Print and shaded views of the part. All mm, measured from the part's lowest x, y and z. A direction names the side the tool comes from. Coordinates: 2 decimals unless noted, no trailing zeros. Order: outer loops, then holes, each group sorted by start corner. A loop starts at its lowest first (then second) coordinate and runs counter-clockwise, first axis right, second up. Notation, with made-up numbers: (33.25, -21.75) -> (51.25, -21.75) arc R21 cw to (51.25, 12.25) -> close; hole circle Ø8 at (80, -32). An arc over 180 degrees is marked (long way). Return JSON: item names as keys, results as strings. Group by question number.
1) Cut at C-C (z = 12.75). Write the cut outline in (x, y), and give its area (3 significant figures).
2) Pull direction X, two halves, no side cores. Call the marked faces 1, 2 and 3: +X half, -X half, draft (parallel to the pull), parting line (faces both ways), or undercut.
3) Probe line 1 (Y direction, x = 12, z = 12.6); line 2 (Y direction, x = 11.5, z = 8); line 3 (Z direction, x = 20, y = 3.3). List the from-to ranges inside material, lowest first.
4) Cut at B-B (z = 7). Write the cut outline in (x, y).
5) Cut at A-A (x = 12). Write the cut outline in (y, z).
6) Flat gauge pins, fed straight in: pin 1 (2.5 mm diameter, centred on x = 4.5, z = 6.5, fed in from +Y); pin 2 (1.5 mm diameter, centred on x = 8, y = 6.5, fed in from -Z); pin 3 (1 mm diameter, centred on x = 3.5, y = 4, fed in from -Z). Where does each tip first touch, or does it go through?
7) Cut at D-D (y = 12). Write the cut outline in (x, z).
8) Which spindle directions (+Z, -Z, +X, -X, +Y, -Y) get a long thin tool onto all of the face, cutting with end or side? Do the marked faces 4, 5 and 6. Say none if no direction does.
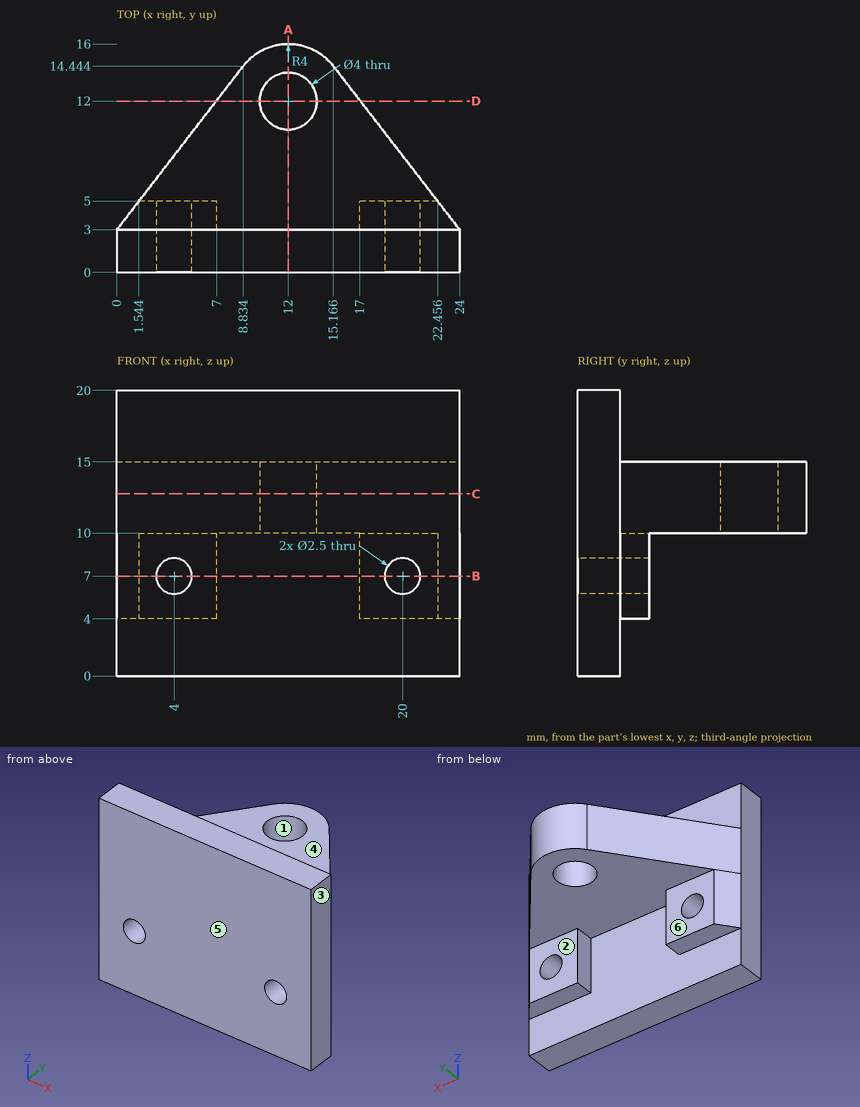
Answers below:
{
 "1": {"outline": "(0, 0) -> (24, 0) -> (24, 3) -> (15.17, 14.44) arc R4 ccw to (8.83, 14.44) -> (0, 3) -> close; hole circle Ø4 at (12, 12)", "area": "240 mm^2"},
 "2": {"face 1": "undercut", "face 2": "draft", "face 3": "+X half"},
 "3": {"line 1": "y = 0 to 10, 14 to 16", "line 2": "y = 0 to 3", "line 3": "z = 4 to 5.75, 8.25 to 15"},
 "4": {"outline": "(0, 0) -> (2.75, 0) -> (2.75, 5) -> (1.54, 5) -> (0, 3) -> close; (5.25, 0) -> (18.75, 0) -> (18.75, 5) -> (17, 5) -> (17, 3) -> (7, 3) -> (7, 5) -> (5.25, 5) -> close; (21.25, 0) -> (24, 0) -> (24, 3) -> (22.46, 5) -> (21.25, 5) -> close"},
 "5": {"outline": "(0, 0) -> (3, 0) -> (3, 10) -> (10, 10) -> (10, 15) -> (3, 15) -> (3, 20) -> (0, 20) -> close; (14, 10) -> (16, 10) -> (16, 15) -> (14, 15) -> close"},
 "6": {"pin 1": "stops at y = 5", "pin 2": "stops at z = 10", "pin 3": "stops at z = 4"},
 "7": {"outline": "(6.95, 10) -> (10, 10) -> (10, 15) -> (6.95, 15) -> close; (14, 10) -> (17.05, 10) -> (17.05, 15) -> (14, 15) -> close"},
 "8": {"face 4": "+Z, +X, -X, +Y", "face 5": "+Z, -Z, +X, -X, -Y", "face 6": "-Z, +X, -X, +Y"}
}
